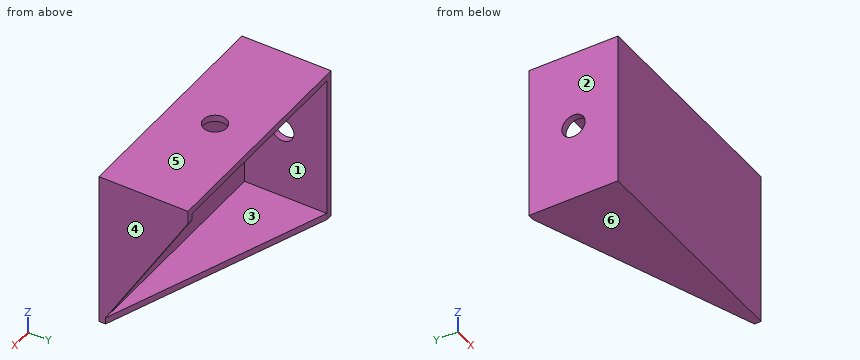
from build123d import *

# Parameters (mm, degrees)
SKETCH_1_W          = 51
SKETCH_1_H          = 35
EXTRUDE_1_DEPTH     = 20
SKETCH_2_W          = 48
SKETCH_2_H          = 32
CUT_EXTRUDE_1_DEPTH = 18.5
SKETCH_3_R          = 2.6
CUT_EXTRUDE_2_DEPTH = 3
SKETCH_4_R          = 2.6
CUT_EXTRUDE_3_DEPTH = 3
CUT_EXTRUDE_4_DEPTH = 1.5
CUT_EXTRUDE_5_DEPTH = 3


with BuildPart() as part:
    # 草图1 → 凸台-拉伸1 (new body)
    with BuildSketch(Plane(origin=(0, 0, 0), x_dir=(1, 0, 0), z_dir=(0, 1, 0))):
        with Locations((25.5, 17.5)):
            Rectangle(SKETCH_1_W, SKETCH_1_H)
    extrude(amount=EXTRUDE_1_DEPTH)

    # 草图2 → 切除-拉伸1 (cut)
    with BuildSketch(Plane(origin=(0, 20, 0), x_dir=(1, 0, 0), z_dir=(0, 1, 0))):
        with Locations((25.5, 17.5)):
            Rectangle(SKETCH_2_W, SKETCH_2_H)
    extrude(amount=-CUT_EXTRUDE_1_DEPTH, mode=Mode.SUBTRACT)

    # 草图3 → 切除-拉伸2 (cut)
    with BuildSketch(Plane.XY):
        with Locations((25.5, 10)):
            Circle(SKETCH_3_R)
    extrude(amount=-CUT_EXTRUDE_2_DEPTH, mode=Mode.SUBTRACT)

    # 草图4 → 切除-拉伸3 (cut)
    with BuildSketch(Plane.ZY):
        with Locations((-17.5, 10)):
            Circle(SKETCH_4_R)
    extrude(amount=-CUT_EXTRUDE_3_DEPTH, mode=Mode.SUBTRACT)

    # 草图5 → 切除-拉伸4 (cut)
    with BuildSketch(Plane(origin=(0, 0, -35), x_dir=(-1, 0, 0), z_dir=(0, 0, -1))):
        Polygon((-51, 20), (-1.5, 20), (-51, 1.5), align=None)
    extrude(amount=-CUT_EXTRUDE_4_DEPTH, mode=Mode.SUBTRACT)

    # 草图6 → 切除-拉伸5 (cut)
    with BuildSketch(Plane(origin=(51, 0, 0), x_dir=(0, 0, -1), z_dir=(1, 0, 0))):
        Polygon((33.5, 20), (33.5, 1.5), (3, 20), align=None)
    extrude(amount=-CUT_EXTRUDE_5_DEPTH, mode=Mode.SUBTRACT)


solid = part.part
The listing builds one solid part. Answer for the finished solid, in the listing's coordinates (mm). Face numbers are marked on the shaded views. A direction names the side the tool comes from. Round coordinates to 2 decimals unless told otherwise and drop trailing zeros. Write each loop counter-clockwise with the first axis right and the second up, starting at its lowest first coordinate (ties: lowest second). Pieces come first, ordered by that corner, then holes. Notation, with made-up numbers: M 59,20.5 L 92,20.5 A24 ccw 92,32.5 Z; hole C 43.25,26 d6. An arc over 180 degrees is marked long. Write each question's results on one line, items separated by ' | '. Start each with the question number.
(1) Find the intervals of material crossed by line 1 (X direction, y = 8.75, z = -4); line 2 (Y direction, x = 25.5, z = -0.3); line 3 (Z direction, x = 14.5, y = 5), in increasing order.
(2) The part is cut by section D-D, the plane z = -25. Write down the section's boundary in (x, y).
(3) The part is cut by section C-C, the plane y = 10. Write down the section's boundary in (x, z).
(4) The part is cut by section B-B, the plane x = 25.5. Write down the section's boundary in (y, z), and give its area (3 significant figures).
(5) The part is cut by section A-A, the plane z = -18. Write down the section's boundary in (x, y).
(6) For the marked faces 1 and 2, determine the directions among +Z, -Z, +X, -X, +Y, -Y from which every point of the face is accessible in a straight line to the end or side of a thin tool.
(7) Determine the mould class of the marked faces 3, 4, 5 and 6 for opening direction Z: +Z half, -Z half, draft (parallel to the pull), parting line (faces both ways), or undercut.
(8) Each of these flat-tipped pins is pushed along its axis until it touches: P1, Ø1.5, axis at x = 6.5, z = -21.5, coming from the +Y side; P2, Ø5.5, axis at x = 36, y = 12, coming from the -Z side; P3, Ø4, axis at x = 25.5, y = 10, coming from the +Z side. Where does it stop, or does it pass through?
Worked answers:
1) line 1: x = 0 to 1.5, 49.5 to 51 | line 2: y = 0 to 7.4, 12.6 to 20 | line 3: z = -35 to -33.5, -1.5 to 0
2) outline: M 0,0 L 51,0 L 51,6.66 L 49.5,6.66 L 49.5,1.5 L 1.5,1.5 L 1.5,20 L 0,20 Z
3) outline: M 0,-35 L 28.26,-35 L 28.26,-33.5 L 1.5,-33.5 L 1.5,-20.1 L 0,-20.1 Z; M 0,-14.9 L 1.5,-14.9 L 1.5,-1.5 L 22.9,-1.5 L 22.9,0 L 0,0 Z; M 28.1,-1.5 L 49.5,-1.5 L 49.5,-19.49 L 51,-19.49 L 51,0 L 28.1,0 Z
4) outline: M 0,-35 L 11.03,-35 L 11.03,-33.5 L 1.5,-33.5 L 1.5,-1.5 L 7.4,-1.5 L 7.4,0 L 0,0 Z; M 12.6,-1.5 L 20,-1.5 L 20,0 L 12.6,0 Z | area: 86.7 mm²
5) outline: M 0,0 L 51,0 L 51,10.9 L 49.5,10.9 L 49.5,1.5 L 1.5,1.5 L 1.5,7.45 L 0,7.45 Z; M 0,12.55 L 1.5,12.55 L 1.5,20 L 0,20 Z
6) face 1: +Y | face 2: +Z, -Z, -X, +Y, -Y
7) face 3: undercut | face 4: draft | face 5: +Z half | face 6: -Z half
8) P1: stops at y = 1.5 | P2: stops at z = -1.5 | P3: stops at z = -33.5
